Verification items for the finished model (mm, model axes). Give positions to 0.01 mm unless a question says otherwise; leave off trailing zeros. Write each loop counter-clockwise with the first axis right and the second up, starting at its lowest first coordinate (ties: lowest second). Pieces come first, ordered by that corner, then holes. Notation, with made-up numbers: (40, 7) -> (58, 7) arc R21 ccw to (58, 43) -> close; hole circle Ø11 at (-6.75, 28.25). An arc over 180 degrees is marked (long way). Write item = value, one per line.
from build123d import *

# Parameters (mm, degrees)
SKETCH1_R           = 59.625
SKETCH1_R_2         = 28.5
BOSS_EXTRUDE1_DEPTH = 2.21
CUT_EXTRUDE2_DEPTH  = 2.21
SKETCH6_R           = 2.5
CUT_EXTRUDE4_DEPTH  = 2.21


with BuildPart() as part:
    # Sketch1 → Boss-Extrude1 (new body)
    with BuildSketch(Plane.XY):
        Circle(SKETCH1_R)
        Circle(SKETCH1_R_2, mode=Mode.SUBTRACT)
    extrude(amount=BOSS_EXTRUDE1_DEPTH)

    # Sketch2 → Cut-Extrude2 (cut)
    with BuildSketch(Plane.XY.offset(2.21)):
        Polygon((-8.874281585, 55.625), (-10.874281585, 58.625), (-8.874281585, 59.625), (9.125718415, 59.625), (11.125718415, 58.625), (9.125718415, 55.625), (9.125718415, 43.625), (-8.874281585, 43.625), align=None)
        Polygon((22.607624736, 51.592526614), (22.547040123, 55.197568848), (24.770188006, 54.957540746), (39.912751597, 45.226006032), (41.054617845, 43.303470864), (37.750188327, 41.8609919), (31.262498517, 31.765949506), (16.119934926, 41.49748422), align=None)
        Polygon((46.911769941, 31.179790564), (48.809835901, 34.245299594), (50.550297923, 32.841450616), (58.027768157, 16.4680747), (57.948966187, 14.233395696), (54.389240175, 14.806414648), (43.473656231, 9.821434492), (35.996185997, 26.194810408), align=None)
        Polygon((56.321759653, 0.867691316), (59.575853655, 2.420389685), (60.281045421, 0.298431963), (57.719378332, -17.518353991), (56.444927213, -19.355682037), (53.760092564, -16.949094638), (41.882235262, -15.241316579), (44.443902351, 2.575469375), align=None)
        Polygon((47.849988626, -29.719893795), (51.426958817, -30.172976848), (50.872986923, -32.339336731), (39.085493712, -45.942829069), (37.02002267, -46.799467484), (36.062495415, -43.323386133), (26.993500522, -35.465057326), (38.780993734, -21.861564987), align=None)
        Polygon((24.186184301, -50.871622616), (26.950367919, -53.186636423), (25.313114529, -54.709594511), (8.042241004, -59.780780534), (5.8415225, -59.384752674), (6.915310776, -55.942808639), (3.534520094, -44.428892956), (20.805393619, -39.357706933), align=None)
        Polygon((-7.156562647, -55.871970699), (-6.08277437, -59.313914733), (-8.283492875, -59.709942593), (-25.5543664, -54.63875657), (-27.19161979, -53.115798483), (-24.427436172, -50.800784675), (-21.04664549, -39.286868992), (-3.775771965, -44.358055015), align=None)
        Polygon((-36.227151521, -43.133362857), (-37.184678776, -46.609444207), (-39.250149819, -45.752805792), (-51.03764303, -32.149313454), (-51.591614923, -29.982953571), (-48.014644732, -29.529870518), (-38.94564984, -21.671541711), (-27.158156629, -35.275034049), align=None)
        Polygon((-53.795875756, -16.700217074), (-56.480710405, -19.106804472), (-57.755161524, -17.269476427), (-60.316828612, 0.547309527), (-59.611636847, 2.669267249), (-56.357542845, 1.11656888), (-44.479685542, 2.82434694), (-41.918018453, -14.992439014), align=None)
        Polygon((-54.284789542, 15.035129632), (-57.844515554, 14.462110681), (-57.923317523, 16.696789684), (-50.445847289, 33.070165601), (-48.705385268, 34.474014578), (-46.807319308, 31.408505549), (-35.891735364, 26.423525393), (-43.369205598, 10.050149476), align=None)
        Polygon((-37.538666206, 41.996928913), (-40.843095724, 43.439407877), (-39.701229476, 45.361943044), (-24.558665885, 55.093477759), (-22.335518002, 55.333505861), (-22.396102615, 51.728463627), (-15.908412806, 41.633421233), (-31.050976397, 31.901886519), align=None)
    extrude(amount=-CUT_EXTRUDE2_DEPTH, mode=Mode.SUBTRACT)

    # Sketch6 → Cut-Extrude4 (cut)
    with BuildSketch(Plane.XY.offset(2.21)):
        with Locations((-13.918677225, 48.02364443)):
            Circle(SKETCH6_R)
        with Locations((14.254405994, 47.925065569)):
            Circle(SKETCH6_R)
        with Locations((37.901816027, 32.610617012)):
            Circle(SKETCH6_R)
        with Locations((49.515667272, 6.942527969)):
            Circle(SKETCH6_R)
        with Locations((45.40864402, -20.92976465)):
            Circle(SKETCH6_R)
        with Locations((26.884697133, -42.157004875)):
            Circle(SKETCH6_R)
        with Locations((-0.174951135, -49.99969392)):
            Circle(SKETCH6_R)
        with Locations((-27.179053654, -41.967833426)):
            Circle(SKETCH6_R)
        with Locations((-45.553998676, -20.61148235)):
            Circle(SKETCH6_R)
        with Locations((-49.465870987, 7.288868739)):
            Circle(SKETCH6_R)
        with Locations((-37.672678769, 32.875055503)):
            Circle(SKETCH6_R)
    extrude(amount=-CUT_EXTRUDE4_DEPTH, mode=Mode.SUBTRACT)


solid = part.part
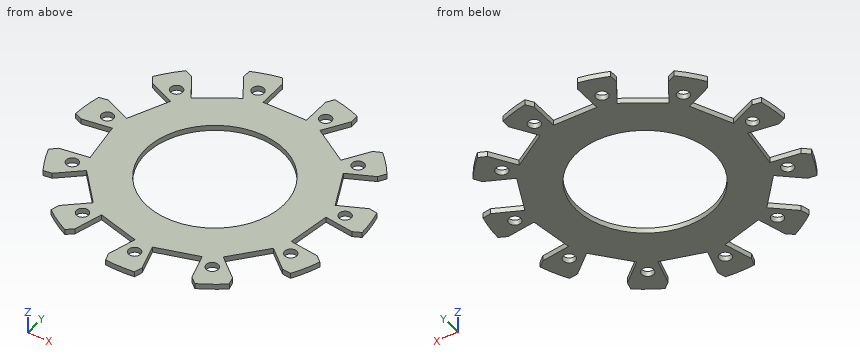
Item 1: Sectioned sample at A-A on y = -4.5. Record the cut outline in (x, z).
Response values:
outline = (-43.43, 0) -> (-28.14, 0) -> (-28.14, 2.21) -> (-43.43, 2.21) -> close; (28.14, 0) -> (43.43, 0) -> (43.43, 2.21) -> (28.14, 2.21) -> close
Item 2: Sectioned sample at B-B on x = 0. Record the cut outline in (y, z) (3 decimals).
Response values:
outline = (-59.625, 0) -> (-52.494, 0) -> (-52.494, 2.21) -> (-59.625, 2.21) -> close; (-47.506, 0) -> (-28.5, 0) -> (-28.5, 2.21) -> (-47.506, 2.21) -> close; (28.5, 0) -> (43.625, 0) -> (43.625, 2.21) -> (28.5, 2.21) -> close
Item 3: Material ranges on line 1 (X direction, y = 38, z = 0.95); line 2 (X direction, y = 37, z = 1.15); line 3 (X direction, y = 33, z = 0.9), recorded low to high.
Response values:
line_1 = -45.95 to -34.97, -21.56 to 21.56, 35.27 to 45.95
line_2 = -46.76 to -34.33, -23.12 to 23.12, 34.63 to 46.76
line_3 = -47.79 to -40.17, -35.18 to -31.76, -29.34 to 29.34, 32.06 to 35.43, 40.37 to 48.04
Item 4: Sectioned sample at C-C on y = 39.5. Record the cut outline in (x, z).
Response values:
outline = (-44.66, 0) -> (-35.93, 0) -> (-35.93, 2.21) -> (-44.66, 2.21) -> close; (-19.23, 0) -> (19.23, 0) -> (19.23, 2.21) -> (-19.23, 2.21) -> close; (36.23, 0) -> (44.66, 0) -> (44.66, 2.21) -> (36.23, 2.21) -> close
Item 5: Go/stop test with flat-tipped pins: P1, Ø4, axis at x = -49.47, y = 7.29, coming from the -Z side; P2, Ø0.7, axis at y = 48.5, z = 1, coming from the -X side; P3, Ø0.7, axis at y = 50.5, z = 1, coming from the +X side. Record where each tip stops, or that it passes through.
Response values:
P1 = through
P2 = -20.55
P3 = 22.13
Item 6: Sectioned sample at D-D on z = 1.2. Give the number of separate pieces and of enclosed holes in the cut face, then the cut area to 3 significant figures.
Response values:
separate_pieces = 1
enclosed_holes = 12
area = 5,210 mm^2
